Read the model definition and answer for the solid it produces. Units are mm, in the model's axes. Give positions to 0.01 mm unless a question says otherwise; leave off trailing zeros. Write each loop counter-clockwise with the first axis right and the second up, starting at its lowest first coordinate (ties: lowest second). Pieces come first, ordered by that corner, then holes. Notation, with made-up numbers: (81, 51) - (95, 51) arc R12 ccw to (95, 73) - close; hole circle Ø3 at (-7.75, -24.75). An arc over 180 degrees is marked (long way). Answer as a JSON object with one key per item and string values. Group by question number.
```python
from build123d import *

# Parameters (mm, degrees)
SKETCH_1_R      = 20.5
SKETCH_1_R_2    = 1.35
SKETCH_1_R_3    = 4
EXTRUDE_1_DEPTH = 4
SKETCH_1_3_R    = 4
SKETCH_1_3_R_2  = 2
EXTRUDE_2_DEPTH = 20
SKETCH_1_4_R    = 22.5
SKETCH_1_4_R_2  = 20.5
EXTRUDE_3_DEPTH = 20
FILLET_1_R      = 5
FILLET_2_R      = 2
CHAMFER_1_SIZE  = 1
SKETCH_2_R      = 4
SKETCH_2_R_2    = 3.05
EXTRUDE_4_DEPTH = 1.5
CHAMFER_2_SIZE  = 0.5


with BuildPart() as part:
    # Sketch 1 → Extrude 1 (new body)
    with BuildSketch(Plane(origin=(0, 0, 0), x_dir=(1, 0, 0), z_dir=(0, 1, 0))):
        Circle(SKETCH_1_R)
        with Locations((0, -8)):
            Circle(SKETCH_1_R_2, mode=Mode.SUBTRACT)
        with Locations((8, 0)):
            Circle(SKETCH_1_R_2, mode=Mode.SUBTRACT)
        with Locations((0, 8)):
            Circle(SKETCH_1_R_2, mode=Mode.SUBTRACT)
        with Locations((-8, 0)):
            Circle(SKETCH_1_R_2, mode=Mode.SUBTRACT)
        Circle(SKETCH_1_R_3, mode=Mode.SUBTRACT)
        with BuildLine():
            ThreePointArc((4, -17.549928775), (12.727922061, -12.727922061), (17.549928775, -4))
            Line((17.549928775, -4), (4, -4))
            Line((4, -4), (4, -17.549928775))
        make_face(mode=Mode.SUBTRACT)
        with BuildLine():
            ThreePointArc((-17.549928775, -4), (-12.727922061, -12.727922061), (-4, -17.549928775))
            Line((-4, -17.549928775), (-4, -4))
            Line((-4, -4), (-17.549928775, -4))
        make_face(mode=Mode.SUBTRACT)
        with BuildLine():
            ThreePointArc((17.549928775, 4), (12.727922061, 12.727922061), (4, 17.549928775))
            Line((4, 17.549928775), (4, 4))
            Line((4, 4), (17.549928775, 4))
        make_face(mode=Mode.SUBTRACT)
        with BuildLine():
            ThreePointArc((-4, 17.549928775), (-12.727922061, 12.727922061), (-17.549928775, 4))
            Line((-17.549928775, 4), (-4, 4))
            Line((-4, 4), (-4, 17.549928775))
        make_face(mode=Mode.SUBTRACT)
    extrude(amount=EXTRUDE_1_DEPTH)

    # Sketch 1_3 → Extrude 2 (add)
    with BuildSketch(Plane(origin=(0, 0, 0), x_dir=(1, 0, 0), z_dir=(0, 1, 0))):
        Circle(SKETCH_1_3_R)
        Circle(SKETCH_1_3_R_2, mode=Mode.SUBTRACT)
    extrude(amount=EXTRUDE_2_DEPTH)

    # Sketch 1_4 → Extrude 3 (add)
    with BuildSketch(Plane(origin=(0, 0, 0), x_dir=(1, 0, 0), z_dir=(0, 1, 0))):
        Circle(SKETCH_1_4_R)
        Circle(SKETCH_1_4_R_2, mode=Mode.SUBTRACT)
    extrude(amount=EXTRUDE_3_DEPTH)

    # Fillet 1
    fillet_1_edges = [part.edges().sort_by_distance(p)[0] for p in [
        (-4, 2, -4),
        (4, 2, -4),
        (-4, 2, 4),
        (4, 2, 4),
    ]]
    fillet(fillet_1_edges, radius=FILLET_1_R)

    # Fillet 2
    fillet_2_edges = [part.edges().sort_by_distance(p)[0] for p in [
        (-17.549928775, 2, -4),
        (-4, 2, -17.549928775),
        (4, 2, -17.549928775),
        (17.549928775, 2, -4),
        (-4, 2, 17.549928775),
        (-17.549928775, 2, 4),
        (17.549928775, 2, 4),
        (4, 2, 17.549928775),
    ]]
    fillet(fillet_2_edges, radius=FILLET_2_R)

    # Chamfer 1
    chamfer_1_edges = [part.edges().sort_by_distance(p)[0] for p in [
        (-22.5, 0, 0),
    ]]
    chamfer(chamfer_1_edges, length=CHAMFER_1_SIZE)

    # Sketch 2 → Extrude 4 (add)
    with BuildSketch(Plane(origin=(0, 20, 0), x_dir=(1, 0, 0), z_dir=(0, 1, 0))):
        Circle(SKETCH_2_R)
        Circle(SKETCH_2_R_2, mode=Mode.SUBTRACT)
    extrude(amount=EXTRUDE_4_DEPTH)

    # Chamfer 2
    chamfer_2_edges = [part.edges().sort_by_distance(p)[0] for p in [
        (-3.05, 21.5, 0),
    ]]
    chamfer(chamfer_2_edges, length=CHAMFER_2_SIZE)


solid = part.part
```
1) Find the intervals of material crossed by line 1 (X direction, y = 13.75, z = 0); line 2 (Z direction, x = 0, y = 0.85), in increasing order. Write a range as [from, to].
2) Find section A-A, the plane z = 0. Give the number of separate pieces and of enclosed holes in the cut face, and give its area (3 significant figures).
3) For a pull along X with two mould halves and no side action, classify faces 1 (the flat face through (4, 0, 0)), 2 (the cylindrical face through (-4.905, 2.028, 16.506)), 3 (the flat face through (12, 2, 4)) as released by +X, released by -X, zero draft, split by the parting line, or undercut.
4) Flat-ended cylindrical pins translate along their axes: pin 1 Ø4.5 at (y, z) = (3, 13.5) entering from -X; pin 2 Ø2 at (x, y) = (11.5, 18.5) entering from -Z; pin 3 Ø1.2 at (y, z) = (2.5, -13) entering from +X. Find the tip coordinate at first contact, or state that the pin passes through.
5) Find section C-C, the plane y = 18.25. Write down the section's boundary in (x, z), and give its area (3 significant figures).
Values follow:
{
 "1": {"line 1": "x = [-22.5, -20.5], [-4, -2], [2, 4], [20.5, 22.5]", "line 2": "z = [-22.35, -9.35], [-6.65, -2], [2, 6.65], [9.35, 22.35]"},
 "2": {"separate pieces": "4", "enclosed holes": "0", "area": "272 mm2"},
 "3": {"face 1": "zero draft", "face 2": "undercut", "face 3": "undercut"},
 "4": {"pin 1": "stops at x = -19.49", "pin 2": "stops at z = -19.9", "pin 3": "stops at x = 18.77"},
 "5": {"outline": "circle Ø45 at (0, 0); circle Ø8 at (0, 0); hole circle Ø41 at (0, 0); hole circle Ø4 at (0, 0)", "area": "308 mm2"}
}
